Read the model definition and answer for the solid it produces. Units are mm, in the model's axes. A direction names the side the tool comes from. Give positions to 0.01 mm unless a question says otherwise; leave off trailing zeros. Order: outer loops, then holes, each group sorted by start corner. A loop starts at its lowest first (then second) coordinate and runs counter-clockwise, first axis right, second up. Notation, with made-up numbers: (81.25, 39.5) - (134.25, 39.5) arc R22 ccw to (134.25, 54.5) - close; hole circle Ø3 at (-6.5, 17). An arc over 180 degrees is marked (long way). Write each question's results on one line, items separated by ' | '.
from build123d import *

# Parameters (mm, degrees)
SKETCH1_W               = 650
SKETCH1_H               = 650
BOSS_EXTRUDE1_DEPTH     = 8
BOSS_EXTRUDE2_DEPTH     = 650
CUT_EXTRUDE2_DEPTH      = 921.277302922
CUT_EXTRUDE2_DEPTH_BACK = 921.277302922
SKETCH4_R               = 16.05
CUT_EXTRUDE1_DEPTH      = 920.932062709
CUT_EXTRUDE1_DEPTH_BACK = 920.932062709
SKETCH2_R               = 210
CUT_EXTRUDE3_DEPTH      = 921.277302998
CUT_EXTRUDE3_DEPTH_BACK = 110
CUT_EXTRUDE4_DEPTH      = 110
CUT_EXTRUDE5_DEPTH      = 920.932062713
CUT_EXTRUDE5_DEPTH_BACK = 920.932062713
SKETCH7_OUTSIDE_W       = 836.056
SKETCH7_OUTSIDE_H       = 836.056
SKETCH7_OUTSIDE_W_2     = 260
SKETCH7_OUTSIDE_H_2     = 231.544504505
BOSS_EXTRUDE3_DEPTH     = 170
SKETCH9_W               = 9.9
SKETCH9_H               = 4
BOSS_EXTRUDE4_DEPTH     = 170
CUT_EXTRUDE6_DEPTH      = 800.941879143
CUT_EXTRUDE6_DEPTH_BACK = 800.941879143
SKETCH10_R              = 210
SKETCH11_W              = 30
SKETCH11_H              = 5
BOSS_EXTRUDE5_DEPTH     = 40
CUT_EXTRUDE7_DEPTH      = 801.144993169
CUT_EXTRUDE7_DEPTH_BACK = 801.144993169
SKETCH13_R              = 2.75
CUT_EXTRUDE8_DEPTH      = 10
SKETCH14_R              = 2.75
CUT_EXTRUDE9_DEPTH      = 10
CUT_EXTRUDE10_DEPTH     = 3
LPATTERN1_COUNT         = 2
LPATTERN1_PITCH         = 40
CUT_EXTRUDE11_DEPTH     = 3
LPATTERN2_COUNT         = 2
LPATTERN2_PITCH         = 40
SKETCH17_R              = 2.15
CUT_EXTRUDE12_DEPTH     = 10
CHAMFER1_SIZE           = 1
SKETCH18_W              = 60.1
SKETCH18_H              = 15.1
CUT_EXTRUDE13_DEPTH     = 3
SKETCH19_R              = 1
CUT_EXTRUDE14_DEPTH     = 10


with BuildPart() as part:
    # Sketch1 → Boss-Extrude1 (new body)
    with BuildSketch(Plane(origin=(0, 0, 0), x_dir=(1, 0, 0), z_dir=(0, 1, 0))):
        with Locations((325, 325)):
            Rectangle(SKETCH1_W, SKETCH1_H)
    extrude(amount=BOSS_EXTRUDE1_DEPTH)

    # Sketch3 → Boss-Extrude2 (add)
    with BuildSketch(Plane.XY):
        Polygon((300, 43.707142143), (350, 43.707142143), (385, 8), (265, 8), align=None)
    extrude(amount=-BOSS_EXTRUDE2_DEPTH)

    # Sketch4 → Cut-Extrude2 (cut, two sides: drawn at the far end of the back side and taken through both)
    with BuildSketch(Plane.XY.offset(-CUT_EXTRUDE2_DEPTH_BACK)):
        with Locations((325, 25)):
            Circle(SKETCH4_R)
    extrude(amount=CUT_EXTRUDE2_DEPTH + CUT_EXTRUDE2_DEPTH_BACK, mode=Mode.SUBTRACT)

    # Sketch2 → Cut-Extrude1 (cut, two sides: drawn at the far end of the back side and taken through both)
    with BuildSketch(Plane(origin=(0, 8, 0), x_dir=(1, 0, 0), z_dir=(0, 1, 0)).offset(-CUT_EXTRUDE1_DEPTH_BACK)):
        with Locations(Location((325, 325, 0), (0, 0, 270))):
            Circle(SKETCH2_R)
    extrude(amount=CUT_EXTRUDE1_DEPTH + CUT_EXTRUDE1_DEPTH_BACK, mode=Mode.SUBTRACT)

    # Sketch5 → Cut-Extrude3 (cut, two sides: drawn at the far end of the back side and taken through both)
    with BuildSketch(Plane.XY.offset(-CUT_EXTRUDE3_DEPTH_BACK)):
        Polygon((300, 43.707142143), (350, 43.707142143), (365.396078824, 28), (350, 28), (350, 8), (300, 8), (300, 28), (284.603921176, 28), align=None)
    extrude(amount=CUT_EXTRUDE3_DEPTH + CUT_EXTRUDE3_DEPTH_BACK, mode=Mode.SUBTRACT)

    # Sketch6 → Cut-Extrude4 (cut)
    with BuildSketch(Plane(origin=(0, 0, -650), x_dir=(-1, 0, 0), z_dir=(0, 0, -1))):
        Polygon((-350, 43.707142143), (-300, 43.707142143), (-284.603921176, 28), (-300, 28), (-300, 8), (-350, 8), (-350, 28), (-365.396078824, 28), align=None)
    extrude(amount=-CUT_EXTRUDE4_DEPTH, mode=Mode.SUBTRACT)

    # Sketch7 outside → Cut-Extrude5 (cut, two sides: drawn at the far end of the back side and taken through both)
    with BuildSketch(Plane(origin=(0, 8, 0), x_dir=(1, 0, 0), z_dir=(0, 1, 0)).offset(-CUT_EXTRUDE5_DEPTH_BACK)):
        with Locations((325, 325)):
            Rectangle(SKETCH7_OUTSIDE_W, SKETCH7_OUTSIDE_H)
        with Locations((325, 570.772252253)):
            Rectangle(SKETCH7_OUTSIDE_W_2, SKETCH7_OUTSIDE_H_2, mode=Mode.SUBTRACT)
    extrude(amount=CUT_EXTRUDE5_DEPTH + CUT_EXTRUDE5_DEPTH_BACK, mode=Mode.SUBTRACT)

    # Sketch8 → Boss-Extrude3 (add)
    with BuildSketch(Plane(origin=(0, 0, -650), x_dir=(-1, 0, 0), z_dir=(0, 0, -1))):
        Polygon((-455, 8), (-455, 28), (-445, 28), (-445, 17), (-435.61916848, 8), align=None)
        Polygon((-195, 8), (-195, 28), (-205, 28), (-205, 17), (-214.38083152, 8), align=None)
    extrude(amount=-BOSS_EXTRUDE3_DEPTH)

    # Sketch9 → Boss-Extrude4 (add)
    with BuildSketch(Plane(origin=(0, 0, -650), x_dir=(-1, 0, 0), z_dir=(0, 0, -1))):
        with Locations((-459.95, 5)):
            Rectangle(SKETCH9_W, SKETCH9_H)
        with Locations((-190.05, 5)):
            Rectangle(SKETCH9_W, SKETCH9_H)
    extrude(amount=-BOSS_EXTRUDE4_DEPTH)

    # Sketch10 → Cut-Extrude6 (cut, two sides: drawn at the far end of the back side and taken through both)
    with BuildSketch(Plane(origin=(0, 8, 0), x_dir=(1, 0, 0), z_dir=(0, 1, 0)).offset(-CUT_EXTRUDE6_DEPTH_BACK)):
        with Locations((325, 325)):
            Circle(SKETCH10_R)
    extrude(amount=CUT_EXTRUDE6_DEPTH + CUT_EXTRUDE6_DEPTH_BACK, mode=Mode.SUBTRACT)

    # Sketch11 → Boss-Extrude5 (add)
    with BuildSketch(Plane(origin=(0, 8, 0), x_dir=(1, 0, 0), z_dir=(0, 1, 0))):
        with Locations((325, 564.5)):
            Rectangle(SKETCH11_W, SKETCH11_H)
    extrude(amount=BOSS_EXTRUDE5_DEPTH)

    # Sketch12 → Cut-Extrude7 (cut, two sides: drawn at the far end of the back side and taken through both)
    with BuildSketch(Plane(origin=(0, 8, 0), x_dir=(1, 0, 0), z_dir=(0, 1, 0)).offset(-CUT_EXTRUDE7_DEPTH_BACK)):
        Polygon((325, 650), (468.244620066, 650), (468.244620066, 575), (178.69132389, 575), (178.69132389, 650), align=None)
    extrude(amount=CUT_EXTRUDE7_DEPTH + CUT_EXTRUDE7_DEPTH_BACK, mode=Mode.SUBTRACT)

    # Sketch13 → Cut-Extrude8 (cut)
    with BuildSketch(Plane(origin=(205, 0, 0), x_dir=(0, 0, -1), z_dir=(1, 0, 0))):
        with Locations((520, 23)):
            Circle(SKETCH13_R)
        with Locations((560, 23)):
            Circle(SKETCH13_R)
    extrude(amount=-CUT_EXTRUDE8_DEPTH, mode=Mode.SUBTRACT)

    # Sketch14 → Cut-Extrude9 (cut)
    with BuildSketch(Plane(origin=(455, 0, 0), x_dir=(0, 0, -1), z_dir=(1, 0, 0))):
        with Locations((560, 23)):
            Circle(SKETCH14_R)
        with Locations((520, 23)):
            Circle(SKETCH14_R)
    extrude(amount=-CUT_EXTRUDE9_DEPTH, mode=Mode.SUBTRACT)

    # Sketch15 → Cut-Extrude10 (cut)
    with BuildSketch(Plane(origin=(205, 0, 0), x_dir=(0, 0, -1), z_dir=(1, 0, 0))):
        Polygon((557.632863896, 27.1), (562.367136104, 27.1), (564.734272207, 23), (562.367136104, 18.9), (557.632863896, 18.9), (555.265727793, 23), align=None)
    cut_extrude10 = extrude(amount=-CUT_EXTRUDE10_DEPTH, mode=Mode.SUBTRACT)

    # LPattern1: Cut-Extrude10 ×2
    with Locations(*[(0, 0, i * LPATTERN1_PITCH) for i in range(1, LPATTERN1_COUNT)]):
        add(cut_extrude10, mode=Mode.SUBTRACT)

    # Sketch16 → Cut-Extrude11 (cut)
    with BuildSketch(Plane.ZY.offset(-445)):
        Polygon((-522.367136104, 27.1), (-517.632863896, 27.1), (-515.265727793, 23), (-517.632863896, 18.9), (-522.367136104, 18.9), (-524.734272207, 23), align=None)
    cut_extrude11 = extrude(amount=-CUT_EXTRUDE11_DEPTH, mode=Mode.SUBTRACT)

    # LPattern2: Cut-Extrude11 ×2
    with Locations(*[(0, 0, -i * LPATTERN2_PITCH) for i in range(1, LPATTERN2_COUNT)]):
        add(cut_extrude11, mode=Mode.SUBTRACT)

    # Sketch17 → Cut-Extrude12 (cut)
    with BuildSketch(Plane(origin=(0, 8, 0), x_dir=(1, 0, 0), z_dir=(0, 1, 0))):
        with Locations(Location((239.38083152, 565, 0), (0, 0, 270))):
            Circle(SKETCH17_R)
        with Locations(Location((410.61916848, 565, 0), (0, 0, 270))):
            Circle(SKETCH17_R)
    extrude(amount=-CUT_EXTRUDE12_DEPTH, mode=Mode.SUBTRACT)

    # Chamfer1
    chamfer1_edges = [part.edges().sort_by_distance(p)[0] for p in [
        (239.38083152, 0, -567.15),
        (239.38083152, 8, -567.15),
        (410.61916848, 8, -567.15),
    ]]
    chamfer(chamfer1_edges, length=CHAMFER1_SIZE)

    # Sketch18 → Cut-Extrude13 (cut)
    with BuildSketch(Plane(origin=(0, 0, 0), x_dir=(-1, 0, 0), z_dir=(0, -1, 0))):
        with Locations((-324.95, 554.45)):
            Rectangle(SKETCH18_W, SKETCH18_H)
    extrude(amount=-CUT_EXTRUDE13_DEPTH, mode=Mode.SUBTRACT)

    # Sketch19 → Cut-Extrude14 (cut)
    with BuildSketch(Plane.XY.offset(-562)):
        with Locations((315.81, 20.26)):
            Circle(SKETCH19_R)
        with Locations((333.81, 20.26)):
            Circle(SKETCH19_R)
        with Locations((333.81, 31.26)):
            Circle(SKETCH19_R)
        with Locations((315.81, 31.26)):
            Circle(SKETCH19_R)
    extrude(amount=-CUT_EXTRUDE14_DEPTH, mode=Mode.SUBTRACT)


solid = part.part
(1) Consider probe 1 along X at (y, z) = (4, -565); probe 2 along X at (y, z) = (20.5, -525); probe 3 along Y at (x, z) = (450.5, -560). Determine where each line is inside the solid, lowest interval first. Write a range as [from, to].
Conclusion:
probe 1: [185.1, 237.23], [241.53, 408.47], [412.77, 464.9] | probe 2: [195, 205], [445, 455] | probe 3: [0, 20.25], [25.75, 28]
(2) The mould has two halves that part along Y. Classify faces 5 (the face through (455, 17, -533)), 6 (the face through (200, 28, -533)), 7 (the face through (451.55, 23.83, -562.62)), 8 (the face through (198.55, 23.83, -522.62)): pulls with the +Y half, pulls with the -Y half, needs draft (parallel to the pull), parting line crosses it, or undercut.
Conclusion:
face 5: needs draft | face 6: pulls with the +Y half | face 7: undercut | face 8: undercut
(3) Each of these flat-tipped pins is pushed along its axis until it touches: pin 1 (3.5 mm diameter, centred on x = 203, z = -520.5, fed in from +Y); pin 2 (3 mm diameter, centred on x = 255.5, z = -533.5, fed in from -Y); pin 3 (10 mm diameter, centred on x = 352.5, y = 34.5, fed in from -Z); pin 4 (4.5 mm diameter, centred on y = 23, z = -520, fed in from -X). Where does it stop, or does it pass through?
Conclusion:
pin 1: y = 28 | pin 2: y = 0 | pin 3: z = -540 | pin 4: through
(4) For faces 1 (the face through (460, 7, -529)), 2 (the face through (325, 28, -562)), 3 (the face through (325, 43.707, -537)), 4 (the face through (205, 23, -537)), determine the directions among +Z, -Z, +X, -X, +Y, -Y from which every point of the face is accessible in a straight line to the end or side of a thin tool.
Conclusion:
face 1: +Z, -Z, +X, +Y | face 2: +Y | face 3: +Z, +X, -X, +Y | face 4: +Z, -Z, +Y
(5) Section D-D (x = 358) is taken. Give the vertices of the cut face in (y, z).
Conclusion:
outline: (0, -575) - (28, -575) - (28, -540) - (35.55, -540) - (35.55, -532.39) - (0, -532.39) - close
(6) Section B-B (z = -511.5) is taken. Give the vertices of the cut face in (x, y), plus the area to 3 significant figures.
Conclusion:
outline: (185.1, 3) - (195, 3) - (195, 0) - (228.47, 0) - (228.47, 8) - (214.38, 8) - (205, 17) - (205, 28) - (195, 28) - (195, 7) - (185.1, 7) - close; (421.53, 0) - (455, 0) - (455, 3) - (464.9, 3) - (464.9, 7) - (455, 7) - (455, 28) - (445, 28) - (445, 17) - (435.62, 8) - (421.53, 8) - close | area: 1,100 mm^2
(7) Section A-A (x = 325) is taken. Give the vertices of the cut face in (y, z), plus the area to 3 significant figures.
Conclusion:
outline: (0, -575) - (8, -575) - (8, -567) - (48, -567) - (48, -562) - (8, -562) - (8, -540) - (8.95, -540) - (8.95, -535) - (0, -535) - (0, -546.9) - (3, -546.9) - (3, -562) - (0, -562) - close; (41.05, -540) - (43.71, -540) - (43.71, -535) - (41.05, -535) - close | area: 493 mm^2
(8) Section C-C (y = 38) is taken. Give the vertices of the cut face in (x, z), plus the area to 3 significant figures.
Conclusion:
outline: (294.41, -540) - (315.59, -540) - (315.59, -534.79) arc R210 cw to (294.41, -532.76) - close; (310, -567) - (340, -567) - (340, -562) - (310, -562) - close; (334.41, -540) - (355.59, -540) - (355.59, -532.76) arc R210 cw to (334.41, -534.79) - close | area: 406 mm^2
